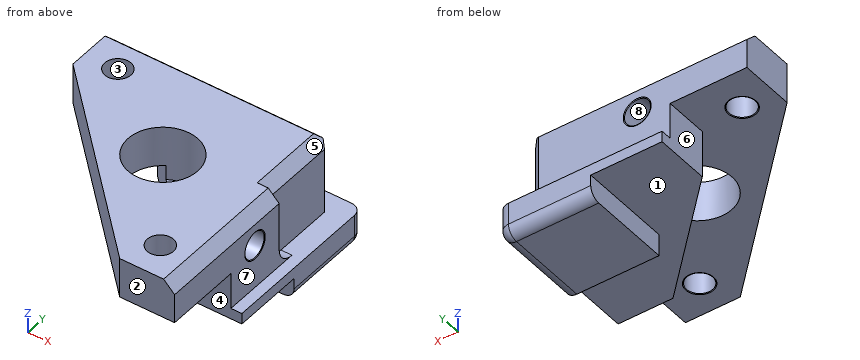
Autodesk Inventor part; units mm, degrees
ref_plane "YZ Plane" through (0, 0, 0) normal (1, 0, 0) x (0, 1, 0)
ref_plane "XZ Plane" through (0, 0, 0) normal (0, 1, 0) x (-1, 0, 0)
ref_plane "XY Plane" through (0, 0, 0) normal (0, 0, 1) x (1, 0, 0)
sketch "Sketch1" plane through (0, 0, 0) normal (0, 0, 1) x (1, 0, 0)
  line L0 (-4.25, 4.25) -> (4.25, 4.25)
  line L1 (4.25, 4.25) -> (4.25, -4.25)
  line L2 (4.25, -4.25) -> (-4.25, -4.25)
  line L3 (-4.25, -4.25) -> (-4.25, 4.25)
  point P0 (0, 0)
  dimension "d0" = 8.5
  dimension "d1" = 8.5
  dimension "d2" = 4.25
  dimension "d3" = 4.25
extrude "Extrusion1" add sketch "Sketch1" along normal blind 3
fillet "Fillet2" radius 1 3 edges at (4.25, 4.25, 1.5) (4.25, 0, 0) (0, 4.25, 0)
sketch "Sketch10" plane through (0, 0, 3) normal (0, 0, 1) x (1, 0, 0)
  line L0 (4.25, 3.25) -> (4.25, -4.25)
  line L1 (-4.25, 4.25) -> (3.25, 4.25)
  line L2 (3.25, 3.25) -> (-17.75, 3.25)
  line L3 (-17.75, 3.25) -> (-17.75, -17.75)
  line L4 (-17.75, -17.75) -> (3.25, -17.75)
  line L5 (3.25, -17.75) -> (3.25, 3.25)
  point P0 (0, 0)
  dimension "d113" = 1
  dimension "d114" = 1
  dimension "d115" = 21
  dimension "d116" = 21
extrude "Extrusion8" add sketch "Sketch10" along normal blind 7
hole "Hole9" at (3.25, -7.75, 7) direction (-1, 0, 0) diameter 2.3876 depth 5 tip angle 118 countersink diameter 2.54 countersink angle 120
hole "Hole10" at (-7.75, 3.25, 7) direction (0, -1, 0) diameter 2.3876 depth 5 tip angle 118 countersink diameter 2.54 countersink angle 120
hole "Hole11" at (-6.25, -6.25, 10) direction (0, 0, -1) diameter 6.35 depth 5
sketch "Sketch11" plane through (0, 0, 3) normal (0, 0, -1) x (-1, 0, 0)
  line L0 (17.75, -17.75) -> (-3.25, -17.75)
  line L1 (17.75, 3.25) -> (17.75, -17.75)
  line L2 (4.25, 3.25) -> (17.75, 3.25)
  line L3 (10.75, 3.25) -> (17.75, 3.25)
  line L4 (17.75, 3.25) -> (17.75, -17.75)
  line L5 (17.75, -17.75) -> (-3.25, -17.75)
  line L6 (-3.25, -17.75) -> (-3.25, -10.75)
  line L7 (-3.25, -10.75) -> (0.75, -10.75)
  line L8 (0.75, -10.75) -> (10.75, -0.75)
  line L9 (10.75, -0.75) -> (10.75, 3.25)
  point P0 (0, 0)
  dimension "d146" = 14
  dimension "d158" = 4
extrude "Extrusion9" cut sketch "Sketch11" against normal blind 3.325
hole "Hole12" at (-0.25, -14.75, 6.325) direction (0, 0, 1) diameter 2.3876 end through all countersink diameter 2.54 countersink angle 120
hole "Hole13" at (-14.75, -0.25, 6.325) direction (0, 0, 1) diameter 2.3876 end through all countersink diameter 2.54 countersink angle 120
chamfer "Chamfer3" distance 16 angle 45 1 edges at (-17.75, -17.75, 8.1625)
hole "Hole14" [suppressed]
sketch "Sketch14" plane through (3.25, -4.25, 3) normal (1, 0, 0) x (0, 0, -1)
  line L0 (0, 7.5) -> (0, 0)
  line L1 (0, 7.5) -> (-7, 7.5)
  line L2 (-7, 7.5) -> (-7, -13.5)
  line L3 (-7, 7.5) -> (0, 7.5)
  line L4 (0, 7.5) -> (0, 1.0875)
  line L5 (-1.5875, -0.5) -> (-7, -0.5)
  line L6 (-7, -0.5) -> (-7, 7.5)
  arc A0 (-1.5875, -0.5) -> (0, 1.0875) centre (-1.5875, 1.0875) ccw
  point P0 (3, 4.25)
  dimension "d180" = 8
  dimension "d181" = 1.5875
extrude "Extrusion10" cut sketch "Sketch14" against normal blind 1
chamfer "Chamfer4" distance 1 angle 45 3 edges at (-7.75, 3.25, 10) (2.25, -0.75, 10) (3.25, -11.25, 10)
chamfer "Chamfer5" distance 1 angle 45 1 edges at (2.25, 3.25, 6.0003)
sketch "Sketch15" plane through (0, 0, 3) normal (0, 0, -1) x (-1, 0, 0)
  line L0 (-3.25, -10.75) -> (0.75, -10.75)
  line L1 (10.75, -0.75) -> (10.75, 3.25)
  line L2 (4.25, 3.25) -> (10.75, 3.25)
  line L3 (4.25, -4.25) -> (4.25, 3.25)
  line L4 (-3.25, -4.25) -> (4.25, -4.25)
  line L5 (-3.25, -10.75) -> (-3.25, -4.25)
  line L6 (4.25, 4.25) -> (10.75, 4.25)
  line L7 (10.75, 4.25) -> (10.75, -0.75)
  line L8 (10.75, -0.75) -> (0.75, -10.75)
  line L9 (0.75, -10.75) -> (-4.25, -10.75)
  line L10 (-4.25, -10.75) -> (-4.25, -4.25)
  line L11 (-4.25, -4.25) -> (4.25, -4.25)
  line L12 (4.25, -4.25) -> (4.25, 4.25)
  point P0 (0, 0)
  dimension "d190" = 1
  dimension "d191" = 1
extrude "Extrusion11" add sketch "Sketch15" along normal blind 1
properties part number "nub_plusZ_3" material "Aluminum-6061"
Geometry: final body of the model. Coordinates: model frame, mm. Face numbers are marked on the shaded views. A direction names the side the tool comes from. Give positions to 0.01 mm unless a question says otherwise; leave off trailing zeros. Write each loop counter-clockwise with the first axis right and the second up, starting at its lowest first coordinate (ties: lowest second). Pieces come first, ordered by that corner, then holes.
(1) Cut plane A-A, the plane y = -0.25. Give the number of separate pieces and of enclosed holes in the cut face, then the cut area to 3 significant figures.
(2) Ray query, line 1 (Z direction, x = -7.75, y = 0); line 2 (X direction, y = -0.25, z = 8.55); line 3 (Y direction, x = 0.2, z = 7). Return the intervals inside material, ascending.
(3) Cut plane D-D, the plane z = 4.25. Return loops of the section in (x, y).
(4) Access query for the marked faces 4, 5, 6, 7 and 8. Directions: +Z, -Z, +X, -X, +Y, -Y. A direction counts if a zero-diameter tool reaches every point of the face in a straight line with its end or side. Return the directions, or none.
(5) First-contact query: P1, Ø0.6, axis at x = 2, z = 6, coming from the +Y side; P2, Ø4, axis at x = -4.5, y = -5, coming from the +Z side; P3, Ø5, axis at x = 0.5, z = 3.5, coming from the -Y side; P4, Ø3, axis at y = -7.75, z = 7, coming from the +X side. Flat tips, straight axial feed; report the tip coordinate or a pass-through.
(6) Mould query, pull axis Y, two halves, no side actions, for the marked faces 1, 2 and 3. Classes: released by +Y, released by -Y, zero draft, split by the parting line, or undercut.
Values follow:
1. separate pieces: 2
1. enclosed holes: 1
1. area: 135 mm2
2. line 1: z = 2 to 5.81, 8.19 to 10
2. line 2: x = -17.75 to -15.94, -13.56 to 2.25
2. line 3: y = -17.75 to -15.86, -13.64 to -8.94, -6.56 to 3.25
3. outline: (-10.75, -0.75) - (-0.75, -10.75) - (3.25, -10.75) - (3.25, -4.71) - (2.25, -4.71) - (2.25, 2.25) - (1.25, 3.25) - (-10.75, 3.25) - close
4. face 4: -Z, +X, -X, -Y
4. face 5: +Z, +X, +Y
4. face 6: -Z, -X, +Y, -Y
4. face 7: +Z, +X, +Y, -Y
4. face 8: +Y
5. P1: stops at y = 2.8
5. P2: stops at z = 10
5. P3: stops at y = -10.75
5. P4: stops at x = 3.25
6. face 1: zero draft
6. face 2: released by -Y
6. face 3: undercut
